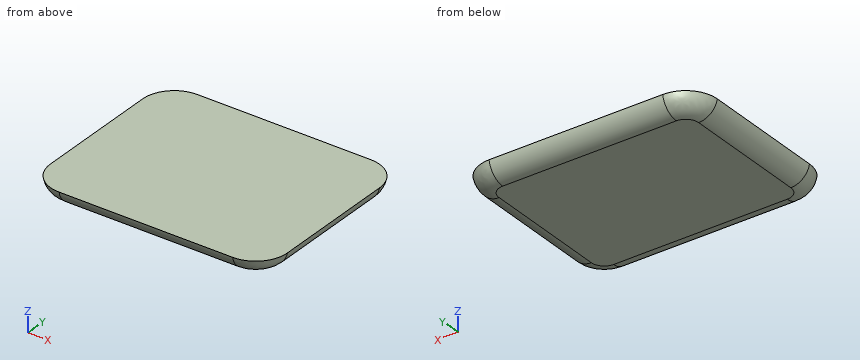
from build123d import *

# Parameters (mm, degrees)
F1_DEPTH     = 25.4
F2_T1_DEPTH  = 279.4
F2_T3_DEPTH  = 203.2
F2_T6_ANGLE  = 90
F2_T8_ANGLE  = 90
F2_T10_ANGLE = 90
F2_T12_ANGLE = 90


# Not quite as in the source:
# - a fillet or chamfer that OpenCascade refuses, or shapes differently, is made with other operations: its cross-section is extruded or revolved along the edge and cut away or added


with BuildPart() as f1:
    # F0 (on Top) → F1 (new body)
    with BuildSketch(Plane.XY):
        with BuildLine():
            Line((-139.7, -152.4), (139.7, -152.4))
            ThreePointArc((139.7, -152.4), (175.6210244843, -137.5210244843), (190.5, -101.6))
            Line((190.5, -101.6), (190.5, 101.6))
            ThreePointArc((190.5, 101.6), (175.6210244843, 137.5210244843), (139.7, 152.4))
            Line((139.7, 152.4), (-139.7, 152.4))
            ThreePointArc((-139.7, 152.4), (-175.6210244843, 137.5210244843), (-190.5, 101.6))
            Line((-190.5, 101.6), (-190.5, -101.6))
            ThreePointArc((-190.5, -101.6), (-175.6210244843, -137.5210244843), (-139.7, -152.4))
        make_face()
    extrude(amount=F1_DEPTH)

    # F2: fillet of radius 30.48 on 1 edges, made by hand

    # F2_s2 → F2_t1 (cut)
    with BuildSketch(Plane.YZ.offset(-139.7)):
        with BuildLine():
            ThreePointArc((-152.4, 25.4), (-142.0210701006, 7.2005154696), (-122.3463147019, 0))
            Line((-122.3463147019, 0), (-152.4, 0))
            Line((-152.4, 0), (-152.4, 25.4))
        make_face()
        with BuildLine():
            ThreePointArc((152.4, 25.4), (142.0210701006, 7.2005154696), (122.3463147019, 0))
            Line((122.3463147019, 0), (152.4, 0))
            Line((152.4, 0), (152.4, 25.4))
        make_face()
    extrude(amount=F2_T1_DEPTH, mode=Mode.SUBTRACT)

    # F2_s4 → F2_t3 (cut)
    with BuildSketch(Plane.XZ.offset(-101.6)):
        with BuildLine():
            ThreePointArc((190.5, 25.4), (180.1210701006, 7.2005154696), (160.4463147019, 0))
            Line((160.4463147019, 0), (190.5, 0))
            Line((190.5, 0), (190.5, 25.4))
        make_face()
        with BuildLine():
            ThreePointArc((-190.5, 25.4), (-180.1210701006, 7.2005154696), (-160.4463147019, 0))
            Line((-160.4463147019, 0), (-190.5, 0))
            Line((-190.5, 0), (-190.5, 25.4))
        make_face()
    extrude(amount=F2_T3_DEPTH, mode=Mode.SUBTRACT)

    # F2_s5 → F2_t6 (revolve, cut)
    with BuildSketch(Plane.XZ.offset(101.6)):
        with BuildLine():
            ThreePointArc((-190.5, 25.4), (-180.1210701006, 7.2005154696), (-160.4463147019, 0))
            Line((-160.4463147019, 0), (-190.5, 0))
            Line((-190.5, 0), (-190.5, 25.4))
        make_face()
    revolve(axis=Axis((-139.7, -101.6, 0), (0, 0, 1)), revolution_arc=F2_T6_ANGLE, mode=Mode.SUBTRACT)

    # F2_s7 → F2_t8 (revolve, cut)
    with BuildSketch(Plane.YZ.offset(139.7)):
        with BuildLine():
            ThreePointArc((-152.4, 25.4), (-142.0210701006, 7.2005154696), (-122.3463147019, 0))
            Line((-122.3463147019, 0), (-152.4, 0))
            Line((-152.4, 0), (-152.4, 25.4))
        make_face()
    revolve(axis=Axis((139.7, -101.6, 0), (0, 0, 1)), revolution_arc=F2_T8_ANGLE, mode=Mode.SUBTRACT)

    # F2_s9 → F2_t10 (revolve, cut)
    with BuildSketch(Plane.XZ.offset(-101.6)):
        with BuildLine():
            ThreePointArc((190.5, 25.4), (180.1210701006, 7.2005154696), (160.4463147019, 0))
            Line((160.4463147019, 0), (190.5, 0))
            Line((190.5, 0), (190.5, 25.4))
        make_face()
    revolve(axis=Axis((139.7, 101.6, 0), (0, 0, 1)), revolution_arc=F2_T10_ANGLE, mode=Mode.SUBTRACT)

    # F2_s11 → F2_t12 (revolve, cut)
    with BuildSketch(Plane.YZ.offset(-139.7)):
        with BuildLine():
            ThreePointArc((152.4, 25.4), (142.0210701006, 7.2005154696), (122.3463147019, 0))
            Line((122.3463147019, 0), (152.4, 0))
            Line((152.4, 0), (152.4, 25.4))
        make_face()
    revolve(axis=Axis((-139.7, 101.6, 0), (0, 0, 1)), revolution_arc=F2_T12_ANGLE, mode=Mode.SUBTRACT)


solid = f1.part
Verification items for the finished model (mm, model axes). Give positions to 0.01 mm unless a question says otherwise; leave off trailing zeros. Loops run counter-clockwise (first coordinate to the right, second up) from the corner with the lowest first, then second, coordinate; pieces in that order, holes last. Notation, with made-up numbers: (57, 81) - (75, 81) arc R29 ccw to (75, 116) - close; hole circle Ø9 at (-5, 34). An arc over 180 degrees is marked (long way). Write each question's results on one line, items separated by ' | '.
1) Sectioned sample at A-A on y = 32. Record the boundary of the cut face in (x, z).
Solution:
outline: (-190.5, 25.4) arc R30.48 ccw to (-160.45, 0) - (160.45, 0) arc R30.48 ccw to (190.5, 25.4) - close
2) Depth check by flat-ended pin: P1, Ø1.5, axis at y = 29.5, z = 21, coming from the -X side; P2, Ø10, axis at y = 37.5, z = 14, coming from the -X side; P3, Ø12, axis at x = -51, z = 12.5, coming from the -Y side. Enter the tip coordinate at first touch or a pass-through.
Solution:
P1: x = -189.65 | P2: x = -188.68 | P3: y = -150.37
3) Material ranges on L1, parallel to Y at x = -145, z = 9; L2, parallel to X at y = -39.5, z = 10.5; L3, parallel to Y at x = -139, z = 11, recorded low to high. Write a range as from..to.
Solution:
L1: -143.64..143.64 | L2: -183.46..183.46 | L3: -145.79..145.79
4) Sectioned sample at B-B on x = -66.5. Record the boundary of the cut face in (y, z), plus the area to 3 significant figures.
Solution:
outline: (-152.4, 25.4) arc R30.48 ccw to (-122.35, 0) - (122.35, 0) arc R30.48 ccw to (152.4, 25.4) - close | area: 7,370 mm2
